from build123d import *

# Parameters (mm, degrees)
SKETCH011_W     = 12.14
SKETCH011_H     = 29
PAD009_DEPTH    = 2.5
CHAMFER002_SIZE = 0.25
SKETCH012_W     = 12.14
SKETCH012_H     = 12.18
PAD010_DEPTH    = 3
SKETCH013_R     = 3.44
PAD011_DEPTH    = 4
PAD008_DEPTH    = 7
CHAMFER001_SIZE = 2
SKETCH004_R     = 28.5
SKETCH004_R_2   = 24.5
PAD002_DEPTH    = 7


with BuildPart() as obj1:
    # Sketch011 → Pad009 (new body)
    with BuildSketch(Plane.XY):
        with Locations((-21.5, 0)):
            Rectangle(SKETCH011_W, SKETCH011_H)
    extrude(amount=PAD009_DEPTH)

    # Chamfer002
    chamfer002_edges = [obj1.edges().sort_by_distance(p)[0] for p in [
        (-15.43, 0, 0),
        (-27.57, 0, 0),
    ]]
    chamfer(chamfer002_edges, length=CHAMFER002_SIZE)

    # Sketch012 → Pad010 (new body)
    with BuildSketch(Plane.XY.offset(2.5)):
        with Locations((-21.5, 0)):
            Rectangle(SKETCH012_W, SKETCH012_H)
    extrude(amount=PAD010_DEPTH)

    # Sketch013 → Pad011 (new body)
    with BuildSketch(Plane.XY.offset(5.5)):
        with Locations((-21.5, 0)):
            Circle(SKETCH013_R)
    extrude(amount=PAD011_DEPTH)


with BuildPart() as chamfer_left_mount:
    # Sketch010 → Pad008 (new body)
    with BuildSketch(Plane.XY):
        with BuildLine():
            ThreePointArc((-14.7, 24.416388), (-28.5, 0), (-14.7, -24.416388))
            Line((-14.7, 24.416388), (-14.7, -24.416388))
        make_face()
    extrude(amount=PAD008_DEPTH)

    # Chamfer001
    chamfer001_edges = [chamfer_left_mount.edges().sort_by_distance(p)[0] for p in [
        (-14.7, 0, 7),
    ]]
    chamfer(chamfer001_edges, length=CHAMFER001_SIZE)


with BuildPart() as cone:
    # Cone → Cone (revolve)
    with BuildSketch(Plane.XZ):
        Polygon((0, 0), (24.5, 0), (28.5, 7), (0, 7), align=None)
    revolve(axis=Axis((0, 0, 0), (0, 0, 1)))


with BuildPart() as cut_left_mount_encoder:
    # Sketch004 → Pad002 (new body)
    with BuildSketch(Plane.XY):
        Circle(SKETCH004_R)
        Circle(SKETCH004_R_2, mode=Mode.SUBTRACT)
    extrude(amount=PAD002_DEPTH)

    # Cut: cut Cone
    add(cone.part, mode=Mode.SUBTRACT)

    # Fusion: union Chamfer (left mount)
    add(chamfer_left_mount.part)

    # Cut001: cut obj1)
    add(obj1.part, mode=Mode.SUBTRACT)


solid = cut_left_mount_encoder.part
The model under review builds one solid part; all positions refer to its coordinate system, in mm. A direction names the side the tool comes from. Coordinates: 2 decimals unless noted, no trailing zeros. Loops run counter-clockwise (first coordinate to the right, second up) from the corner with the lowest first, then second, coordinate; pieces in that order, holes last.
(1) Draft analysis for pull direction Y (two halves, no side actions). For faces 1 (the flat face through (-25.3, 0.3, 7)), 2 (the flat face through (-14.7, 0, 2)), state which applies: +Y half, -Y half, draft (parallel to the pull), parting line (faces both ways), or undercut.
Determined:
face 1: draft
face 2: undercut
(2) Consider section B-B, the plane z = 1.5. Give the boundary of the cut face in (x, y), plus the area to 3 significant figures.
Determined:
outline: (-27.57, -7.22) - (-27.57, 7.22) arc R28.5 ccw to start; (-24.54, -14.5) arc R28.5 ccw (long way) to (-24.54, 14.5) - (-15.43, 14.5) - (-15.43, -14.5) - close; hole (-14.7, -20.66) arc R25.36 ccw (long way) to (-14.7, 20.66) - close
area: 508 mm2
(3) Consider section C-C, the plane x = 0. Give the boundary of the cut face in (y, z).
Determined:
outline: (-28.5, 0) - (-24.5, 0) - (-28.5, 7) - close; (24.5, 0) - (28.5, 0) - (28.5, 7) - close
(4) Consider section A-A, the plane y = 0. Give the boundary of the cut face in (x, z), plus the area to 3 significant figures.
Determined:
outline: (-28.5, 0) - (-27.32, 0) - (-27.57, 0.25) - (-27.57, 5.5) - (-24.94, 5.5) - (-24.94, 7) - (-28.5, 7) - close; (-18.06, 5.5) - (-15.43, 5.5) - (-15.43, 0.25) - (-15.68, 0) - (-14.7, 0) - (-14.7, 5) - (-16.7, 7) - (-18.06, 7) - close; (24.5, 0) - (28.5, 0) - (28.5, 7) - close
area: 31.6 mm2
(5) Wall thickness on L1, parallel to X at y = 0, z = 6.15; L2, parallel to X at y = 0, z = 5.85; L3, parallel to X at y = -10.5, z = 4.5: over which ranges is each line inside the solid? List them lowest first.
Determined:
L1: x = -28.5 to -24.94, -18.06 to -15.85, 28.01 to 28.5
L2: x = -28.5 to -24.94, -18.06 to -15.55, 27.84 to 28.5
L3: x = -26.5 to -14.7, 24.95 to 26.5
(6) Insertion check: P1, Ø3, axis at x = -22.5, z = 1.5, coming from the +Y side; P2, Ø11, axis at x = -21.5, y = 0, coming from the -Z side; P3, Ø6.5, axis at x = -21, y = 9, coming from the -Z side. Each pin has a flat end and moves straight along its axis. Give the tip position at first contact, or say it passes through.
Determined:
P1: stops at y = 19.27
P2: stops at z = 5.5
P3: stops at z = 2.5
(7) Tool access review of faces 3 (the flat face through (-15.7, 0.3, 6)), 4 (the flat face through (20, 15, 0)), 5 (the flat face through (-27.57, 0, 3)): name each direction out of +Z, -Z, +X, -X, +Y, -Y from which nothing blocks a thin tool from reaching the whole face with its end or side.
Determined:
face 3: +Z
face 4: -Z, +X, -X, +Y, -Y
face 5: none
